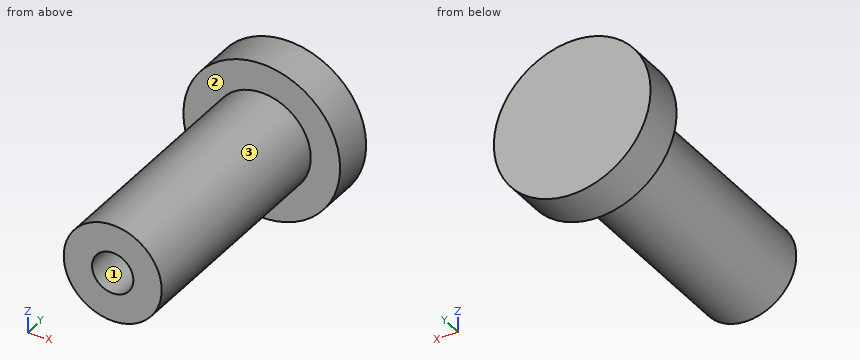
from build123d import *

# Parameters (mm, degrees)
SKETCH1_R           = 3.96875
BOSS_EXTRUDE1_DEPTH = 20
SKETCH2_R           = 1.675
CUT_EXTRUDE1_DEPTH  = 12
SKETCH4_R           = 6.35
BOSS_EXTRUDE2_DEPTH = 2.54
SKETCH6_R           = 6.35
BOSS_EXTRUDE3_DEPTH = 3.35


with BuildPart() as part:
    # Sketch1 → Boss-Extrude1 (new body)
    with BuildSketch(Plane(origin=(0, 0, 0), x_dir=(1, 0, 0), z_dir=(0, 1, 0))):
        Circle(SKETCH1_R)
    extrude(amount=BOSS_EXTRUDE1_DEPTH)

    # Sketch2 → Cut-Extrude1 (cut)
    with BuildSketch(Plane.XZ):
        Circle(SKETCH2_R)
    extrude(amount=-CUT_EXTRUDE1_DEPTH, mode=Mode.SUBTRACT)

    # Sketch4 → Boss-Extrude2 (add)
    with BuildSketch(Plane(origin=(0, 20, 0), x_dir=(1, 0, 0), z_dir=(0, 1, 0))):
        Circle(SKETCH4_R)
    extrude(amount=BOSS_EXTRUDE2_DEPTH)

    # Sketch6 → Boss-Extrude3 (add)
    with BuildSketch(Plane(origin=(0, 22.54, 0), x_dir=(1, 0, 0), z_dir=(0, 1, 0))):
        Circle(SKETCH6_R)
    extrude(amount=-BOSS_EXTRUDE3_DEPTH)


solid = part.part
The listing builds one solid part. Answer for the finished solid, in the listing's coordinates (mm). Face numbers are marked on the shaded views. Round coordinates to 2 decimals unless told otherwise and drop trailing zeros. Order: outer loops, then holes, each group sorted by start corner. A loop starts at its lowest first (then second) coordinate and runs counter-clockwise, first axis right, second up. Notation, with made-up numbers: (3.5, 84.25) -> (46.5, 84.25) arc R22 cw to (46.5, 114.25) -> close; hole circle Ø2 at (86, 47.5). An arc over 180 degrees is marked (long way). One line per item, written item: value.
Item 1: Straight lines are drawn through the part: L1, parallel to Z at x = 0, y = 3 (3 decimals); L2, parallel to X at y = 1.75, z = -1.5; L3, parallel to Y at x = 4.75, z = 1. For each, find the intervals that lie inside material, in ascending order.
Taken from the geometry:
L1: z = -3.969 to -1.675, 1.675 to 3.969
L2: x = -3.67 to -0.75, 0.75 to 3.67
L3: y = 19.19 to 22.54
Item 2: Find section B-B, the plane x = 2.75. Give the vertices of the cut face in (y, z), then the cut area to 3 significant figures.
Taken from the geometry:
outline: (0, -2.86) -> (19.19, -2.86) -> (19.19, -5.72) -> (22.54, -5.72) -> (22.54, 5.72) -> (19.19, 5.72) -> (19.19, 2.86) -> (0, 2.86) -> close
area: 148 mm2
Item 3: For a pull along Z with two mould halves and no side action, classify the marked faces 1, 2 and 3 as released by +Z, released by -Z, zero draft, split by the parting line, or undercut.
Taken from the geometry:
face 1: undercut
face 2: zero draft
face 3: split by the parting line
Item 4: Given P1, Ø4, axis at x = -1.5, y = 4, coming from the +Z side; P2, Ø1, axis at y = 12.5, z = -1, coming from the +X side; P3, Ø4, axis at x = -0.5, y = 4.5, coming from the -Z side, each flat-ended and moving along its own axis, determine where each tip first touches the part or whether it passes through.
Taken from the geometry:
P1: stops at z = 3.97
P2: stops at x = 3.94
P3: stops at z = -3.97
Item 5: Find section A-A, the plane z = 0. Give the vertices of the cut face in (x, y) (3 decimals), then the cut area to 3 significant figures.
Taken from the geometry:
outline: (-6.35, 19.19) -> (-3.969, 19.19) -> (-3.969, 0) -> (-1.675, 0) -> (-1.675, 12) -> (1.675, 12) -> (1.675, 0) -> (3.969, 0) -> (3.969, 19.19) -> (6.35, 19.19) -> (6.35, 22.54) -> (-6.35, 22.54) -> close
area: 155 mm2
Item 6: Find section C-C, the plane y = 12.25. Give the vertices of the cut face in (x, z), then the cut area to 3 significant figures.
Taken from the geometry:
outline: circle Ø7.94 at (0, 0)
area: 49.5 mm2
